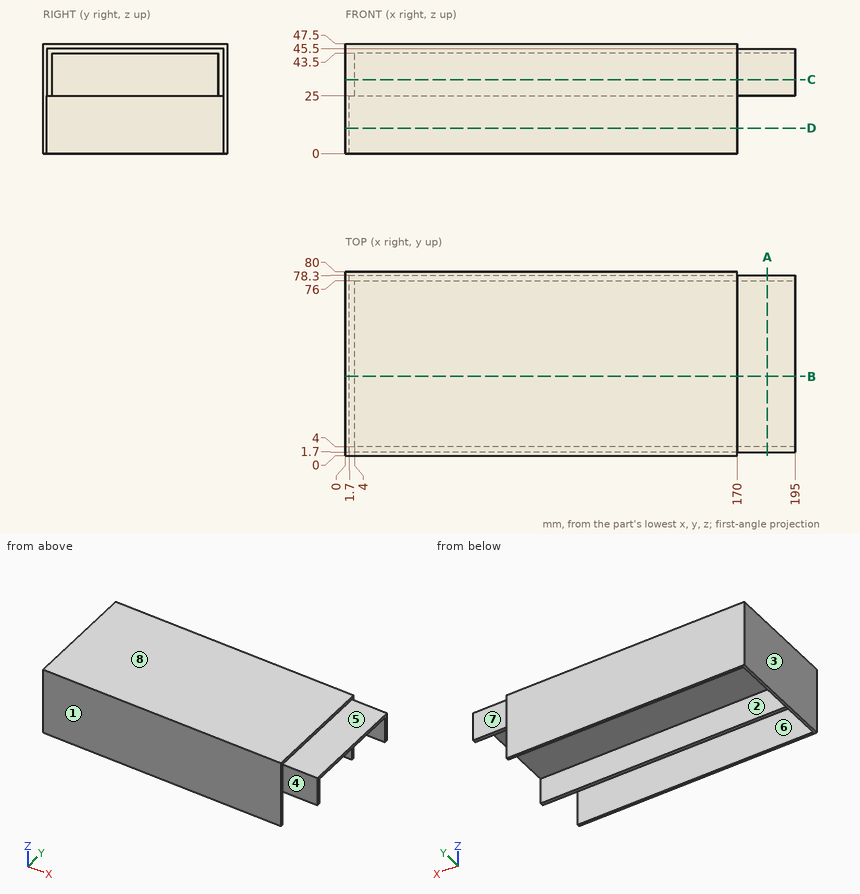
Geometry: see drawing. Coordinates: mm, zero at the bounding-box minimum. A direction names the side the tool comes from. Coordinates: 2 decimals unless noted, no trailing zeros. Loops run counter-clockwise (first coordinate to the right, second up) from the corner with the lowest first, then second, coordinate; pieces in that order, holes last. Notation, with made-up numbers: (68, 38.25) - (87, 38.25) arc R14 ccw to (87, 48.25) - close; hole circle Ø2 at (60, 23.25). An arc over 180 degrees is marked (long way). Answer in a Markdown table with one row per item.
(1) Material intervals for L1, parallel to Y at x = 96, z = 8; L2, parallel to Y at x = 91, z = 41; L3, parallel to X at y = 33, z = 40, sorted ascending. Write a range as from..to.
Model answer:
| item | result |
|---|---|
| L1 | y = 0..1.7, 78.3..80 |
| L2 | y = 0..4, 76..80 |
| L3 | x = 0..4 |
(2) Cut plane D-D on z = 11. Output: boundary loops of the cut face in (x, y).
Model answer:
| item | result |
|---|---|
| outline | (0, 0) - (170, 0) - (170, 1.7) - (1.7, 1.7) - (1.7, 78.3) - (170, 78.3) - (170, 80) - (0, 80) - close |
(3) Pin query (flat end, axial travel): P1, Ø3, axis at x = 158, y = 51, coming from the -Z side; P2, Ø15, axis at y = 32.5, z = 34.5, coming from the +X side; P3, Ø4, axis at y = 61, z = 10, coming from the +X side. Return the tip coordinate at first contact, or that it passes through.
Model answer:
| item | result |
|---|---|
| P1 | stops at z = 43.5 |
| P2 | stops at x = 4 |
| P3 | stops at x = 1.7 |
(4) Set-up query: the marked faces 4, 5, 6, 7 and 8. Return all of +Z, -Z, +X, -X, +Y, -Y with unobstructed straight access to the full face (end or side cutting, diameter ignored); none if empty.
Model answer:
| item | result |
|---|---|
| face 4 | +Z, -Z, +X, -Y |
| face 5 | +Z, +X, +Y, -Y |
| face 6 | -Z, +X |
| face 7 | +Z, -Z, +X, +Y |
| face 8 | +Z, +X, -X, +Y, -Y |
(5) Cut plane C-C on z = 32. Output: boundary loops of the cut face in (x, y).
Model answer:
| item | result |
|---|---|
| outline | (0, 0) - (170, 0) - (170, 1.7) - (195, 1.7) - (195, 4) - (4, 4) - (4, 76) - (195, 76) - (195, 78.3) - (170, 78.3) - (170, 80) - (0, 80) - close |
(6) Cut plane A-A on x = 183. Output: boundary loops of the cut face in (y, z), plus the area to 3 significant figures.
Model answer:
| item | result |
|---|---|
| outline | (1.7, 25) - (4, 25) - (4, 43.5) - (76, 43.5) - (76, 25) - (78.3, 25) - (78.3, 45.5) - (1.7, 45.5) - close |
| area | 238 mm² |
(7) Mould query, pull axis Y, two halves, no side actions, for the marked faces 1, 2 and 3. Classes: pulls with the +Y half, pulls with the -Y half, needs draft (parallel to the pull), parting line crosses it, or undercut.
Model answer:
| item | result |
|---|---|
| face 1 | pulls with the -Y half |
| face 2 | undercut |
| face 3 | needs draft |
(8) Cut plane B-B on y = 34.5. Output: boundary loops of the cut face in (x, z), plus the area to 4 significant figures.
Model answer:
| item | result |
|---|---|
| outline | (0, 0) - (1.7, 0) - (1.7, 25) - (4, 25) - (4, 43.5) - (195, 43.5) - (195, 45.5) - (170, 45.5) - (170, 47.5) - (0, 47.5) - close |
| area | 846.5 mm² |
